```python
from build123d import *

# Parameters (mm, degrees)
SKETCH2_W           = 9
SKETCH2_H           = 8
BOSS_EXTRUDE1_DEPTH = 180
SKETCH3_R           = 1.5
CUT_EXTRUDE1_DEPTH  = 9
SKETCH4_W           = 8
SKETCH4_H           = 7
CUT_EXTRUDE2_DEPTH  = 181
SKETCH5_R           = 3.5
CUT_EXTRUDE3_DEPTH  = 10


with BuildPart() as part:
    # Sketch2 → Boss-Extrude1 (new body)
    with BuildSketch(Plane.XY):
        Rectangle(SKETCH2_W, SKETCH2_H)
    extrude(amount=BOSS_EXTRUDE1_DEPTH)

    # Sketch3 → Cut-Extrude1 (cut, through all)
    with BuildSketch(Plane(origin=(0, 4, 0), x_dir=(1, 0, 0), z_dir=(0, 1, 0))):
        with Locations((0, -2.500384155)):
            Circle(SKETCH3_R)
    extrude(amount=-CUT_EXTRUDE1_DEPTH, mode=Mode.SUBTRACT)

    # Sketch4 → Cut-Extrude2 (cut, through all)
    with BuildSketch(Plane.XY):
        Rectangle(SKETCH4_W, SKETCH4_H)
    extrude(amount=CUT_EXTRUDE2_DEPTH, mode=Mode.SUBTRACT)

    # Sketch5 → Cut-Extrude3 (cut, through all)
    with BuildSketch(Plane(origin=(4.5, 0, 0), x_dir=(0, 0, -1), z_dir=(1, 0, 0))):
        with Locations((-175.980500671, 0)):
            Circle(SKETCH5_R)
    extrude(amount=-CUT_EXTRUDE3_DEPTH, mode=Mode.SUBTRACT)


solid = part.part
```
Input: part model. Units: mm. Frame: model coordinates. A direction names the side the tool comes from. Round coordinates to 2 decimals unless told otherwise and drop trailing zeros. Write each loop counter-clockwise with the first axis right and the second up, starting at its lowest first coordinate (ties: lowest second). Pieces come first, ordered by that corner, then holes. Notation, with made-up numbers: (53, 8.5) - (72, 8.5) arc R18 ccw to (72, 36.5) - close; hole circle Ø11 at (67, 34.25). An arc over 180 degrees is marked (long way). Write item = value, one per line.
(1) Access query for faces 4 (the flat face through (4, 0, 87)), 5 (the flat face through (-4.5, 0, 89)). Directions: +Z, -Z, +X, -X, +Y, -Y. A direction counts if a zero-diameter tool reaches every point of the face in a straight line with its end or side. Return the directions, or none.
Geometry check:
face_4 = +Z, -Z
face_5 = +Z, -Z, -X, +Y, -Y
(2) Pull-direction query (X, two-part tool) for faces 1 (the flat face through (4.5, 0, 89)), 2 (the flat face through (4, -0.3, 179.8)), 3 (the flat face through (0, -4, 89)); classes: +X half, -X half, draft (parallel to the pull), parting line (faces both ways), or undercut.
Geometry check:
face_1 = +X half
face_2 = undercut
face_3 = draft
(3) Section query B-B on z = 108.5. Output: boundary loops of the cut face in (x, y), then the cut area to 3 significant figures.
Geometry check:
outline = (-4.5, -4) - (4.5, -4) - (4.5, 4) - (-4.5, 4) - close; hole (-4, -3.5) - (4, -3.5) - (4, 3.5) - (-4, 3.5) - close
area = 16.0 mm^2
(4) Section query C-C on y = 0. Output: boundary loops of the cut face in (x, z).
Geometry check:
outline = (-4.5, 0) - (-4, 0) - (-4, 172.48) - (-4.5, 172.48) - close; (-4.5, 179.48) - (-4, 179.48) - (-4, 180) - (-4.5, 180) - close; (4, 0) - (4.5, 0) - (4.5, 172.48) - (4, 172.48) - close; (4, 179.48) - (4.5, 179.48) - (4.5, 180) - (4, 180) - close
(5) Contact query for flat-ended pins moving along their axis: pin 1 Ø1.2 at (y, z) = (0, 178) entering from +X; pin 2 Ø3.5 at (x, z) = (0, 2.5) entering from -Y. Output: stop coordinate, or through.
Geometry check:
pin_1 = through
pin_2 = -4
(6) Material intervals for probe 1 along Y at (x, z) = (2, 23); probe 2 along Z at (x, y) = (0, 3.7); probe 3 along X at (y, z) = (2, 67.5), sorted ascending.
Geometry check:
probe_1 = -4 to -3.5, 3.5 to 4
probe_2 = 0 to 1, 4 to 180
probe_3 = -4.5 to -4, 4 to 4.5
(7) Section query A-A on x = 0. Output: boundary loops of the cut face in (y, z).
Geometry check:
outline = (-4, 0) - (-3.5, 0) - (-3.5, 1) - (-4, 1) - close; (-4, 4) - (-3.5, 4) - (-3.5, 180) - (-4, 180) - close; (3.5, 0) - (4, 0) - (4, 1) - (3.5, 1) - close; (3.5, 4) - (4, 4) - (4, 180) - (3.5, 180) - close
